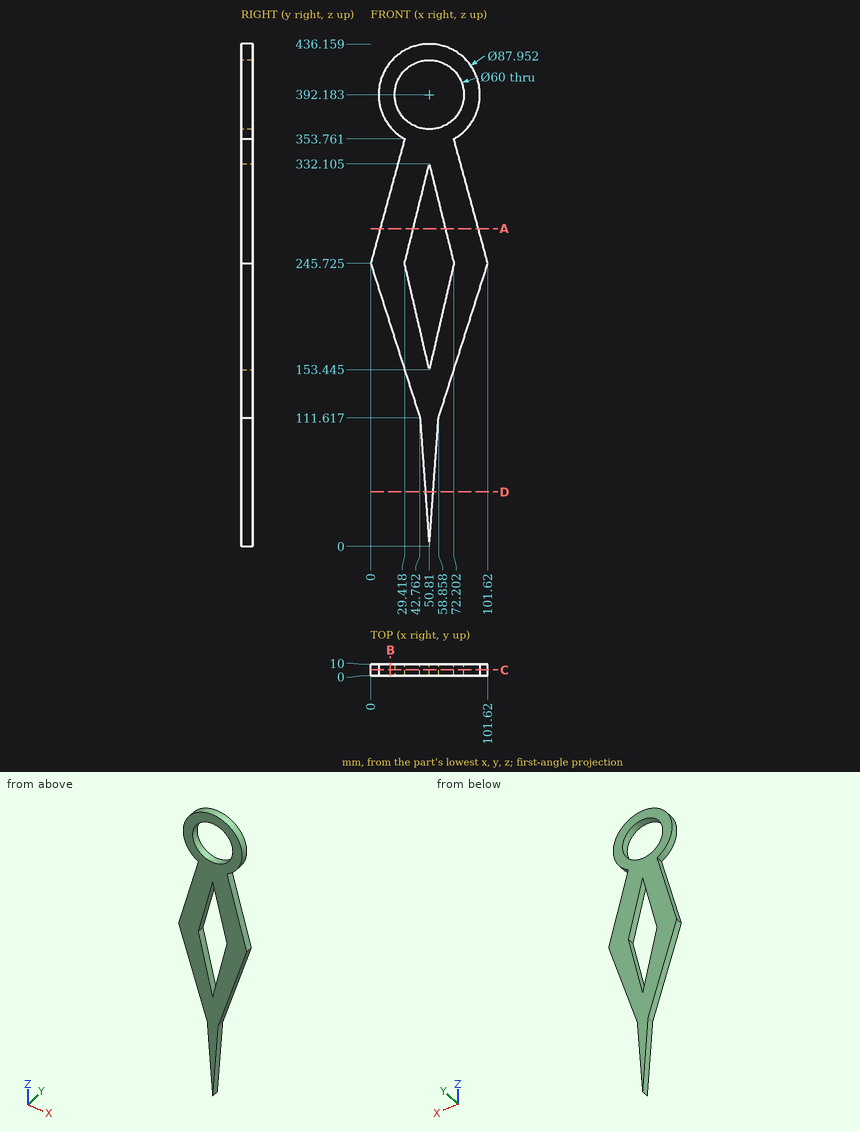
Geometry check sheet. Reference: drawing and pictorial views, mm from the part's lowest x, y, z. Round coordinates to 2 decimals unless told otherwise and drop trailing zeros. Loops run counter-clockwise (first coordinate to the right, second up) from the corner with the lowest first, then second, coordinate; pieces in that order, holes last. Notation, with made-up numbers: (7.5, 48.5) - (64.5, 48.5) arc R21 ccw to (64.5, 54.5) - close; hole circle Ø11 at (4, -12). An arc over 180 degrees is marked (long way). Answer in a Markdown table with one row per item. Add a question column.
Q1. Section check A-A on z = 276. Enter the section's corners in (x, y) (1 decimal).
Q2. Section check B-B on x = 17. Enter the section's corners in (y, z), plus the area to 3 significant figures.
Q3. Section check D-D on z = 47.5. Enter the section's corners in (x, y) (1 decimal), plus the area to 3 significant figures.
Q4. Gauge pin test, flat ends, axial feed: pin 1 (1.5 mm diameter, centred on x = 62, y = 1.5, fed in from +Z); pin 2 (6 mm diameter, centred on y = 7, z = 83, fed in from +X); pin 3 (5 mm diameter, centred on x = 16.5, y = 6.5, fed in from +Z). Record the tip position at first contact, or that the pin passes through.
Q5. Section check C-C on y = 5.25. Enter the section's corners in (x, z) (1 decimal).
Q6. Material ranges on line 1 (X direction, y = 9.75, z = 204) (1 decimal); line 2 (X direction, y = 9.75, z = 286); line 3 (X direction, y = 9, z = 140), recorded low to high.
Found:
| question | item | result |
|---|---|---|
| 1 | outline | (8.2, 0) - (36.9, 0) - (36.9, 10) - (8.2, 10) - close; (64.7, 0) - (93.4, 0) - (93.4, 10) - (64.7, 10) - close |
| 2 | outline | (0, 192.41) - (10, 192.41) - (10, 308.16) - (0, 308.16) - close; (0, 364.06) - (10, 364.06) - (10, 420.3) - (0, 420.3) - close |
| 2 | area | 1,720 mm² |
| 3 | outline | (47.4, 0) - (54.2, 0) - (54.2, 10) - (47.4, 10) - close |
| 3 | area | 68.5 mm² |
| 4 | pin 1 | stops at z = 434.9 |
| 4 | pin 2 | stops at x = 57.01 |
| 4 | pin 3 | stops at z = 422.55 |
| 5 | outline | (0, 245.7) - (42.8, 111.6) - (50.8, 0) - (58.9, 111.6) - (101.6, 245.7) - (72.2, 353.8) arc R44 ccw (long way) to (29.4, 353.8) - close; hole circle Ø60 at (50.8, 392.2); hole (29.4, 245.7) - (50.8, 153.4) - (72.2, 245.7) - (50.8, 332.1) - close |
| 6 | line 1 | x = 13.3 to 39.1, 62.5 to 88.3 |
| 6 | line 2 | x = 10.97 to 39.39, 62.23 to 90.65 |
| 6 | line 3 | x = 33.71 to 67.91 |
